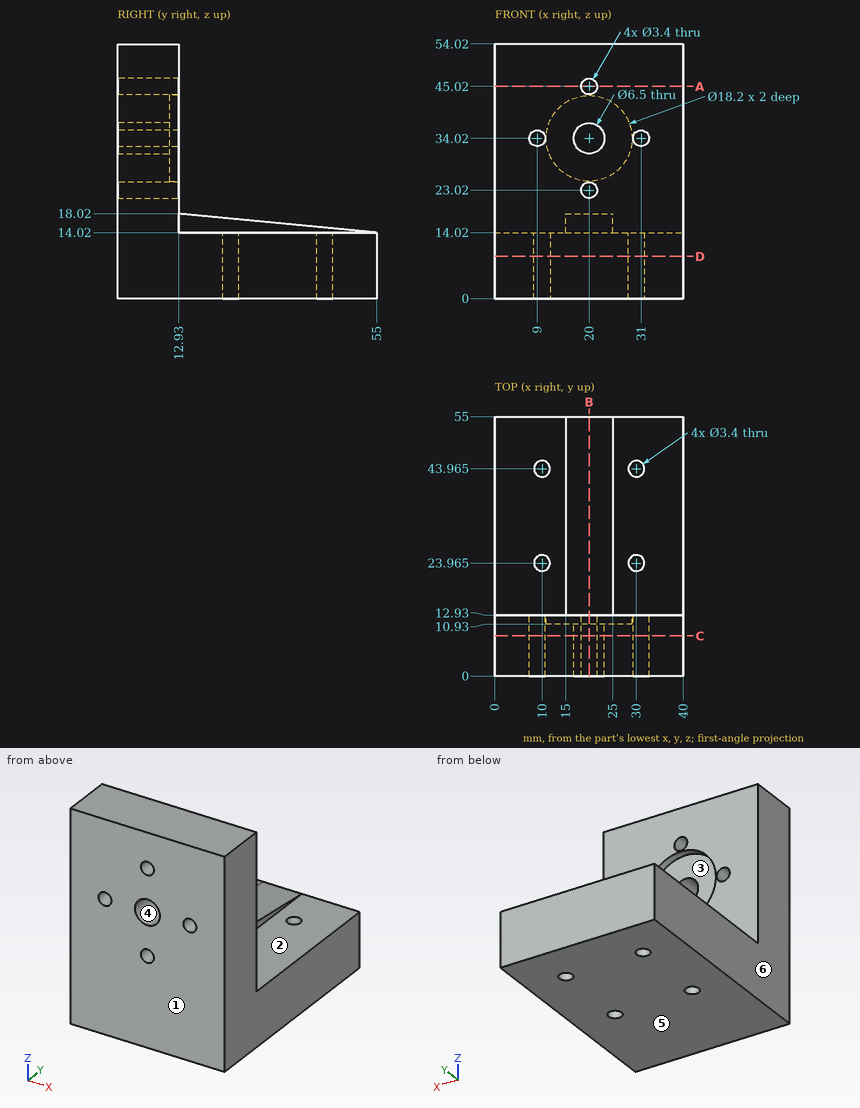
Design review of the part shown in the three views and the two pictorial views. Dimensions are in mm from the part's minimum x, y and z. A direction names the side the tool comes from. Round coordinates to 2 decimals unless told otherwise and drop trailing zeros. Write each loop counter-clockwise with the first axis right and the second up, starting at its lowest first coordinate (ties: lowest second). Pieces come first, ordered by that corner, then holes. Notation, with made-up numbers: M 70.25,16.25 L 75.25,16.25 A26 ccw 75.25,35.25 Z; hole C 16,-12 d3. An arc over 180 degrees is marked long. One line per item, written item: value. Start each with the question number.
1. For the marked faces 1, 2 and 3, list the 3-axis set-ups (+Z, -Z, +X, -X, +Y, -Y) from which the entire face can be reached by the end or side of a thin tool; tool diameter is ignored.
2. To check wall thickness, follow probe 1 along Y at (x, z) = (30, 8) (3 decimals); probe 2 along X at (y, z) = (5.25, 45.02); probe 3 along Y at (x, z) = (29.5, 36.5). State the ranges of each line that lie inside material, in increasing order. Write a range as from..to.
3. Clearance check with flat-ended pins moving along their axes: P1, Ø4, axis at x = 19.5, y = 23.5, coming from the +Z side; P2, Ø4, axis at x = 20, z = 23.02, coming from the +Y side; P3, Ø1, axis at x = 21.5, z = 30, coming from the +Y side. State where each tip first meets the part, or that it passes through.
4. Take a section at B-B on x = 20. State the section outline as (y, z) points, then the cut area to 3 significant figures.
5. Take a section at D-D on z = 9. State the section outline as (x, y) points (3 decimals).
6. Take a section at C-C on y = 8.5. State the section outline as (x, z) points, then the cut area to 3 significant figures.
7. Take a section at A-A on z = 45.02. State the section outline as (x, y) points, then the cut area to 3 significant figures.
8. Draft analysis for pull direction X (two halves, no side actions). For the marked faces 4, 5 and 6, state which applies: pulls with the +X half, pulls with the -X half, needs draft (parallel to the pull), parting line crosses it, or undercut.
Computed:
1. face 1: +Z, -Z, +X, -X, -Y
1. face 2: +Z, +X, +Y
1. face 3: +Y
2. probe 1: y = 0..22.265, 25.665..42.265, 45.665..55
2. probe 2: x = 0..18.3, 21.7..40
2. probe 3: y = 0..12.93
3. P1: stops at z = 17.21
3. P2: stops at y = 12.93
3. P3: stops at y = 10.93
4. outline: M 0,0 L 55,0 L 55,14.02 L 12.93,18.02 L 12.93,21.32 L 0,21.32 Z; M 0,24.72 L 12.93,24.72 L 12.93,24.92 L 10.93,24.92 L 10.93,30.77 L 0,30.77 Z; M 0,37.27 L 10.93,37.27 L 10.93,43.12 L 12.93,43.12 L 12.93,43.32 L 0,43.32 Z; M 0,46.72 L 12.93,46.72 L 12.93,54.02 L 0,54.02 Z
4. area: 1,180 mm²
5. outline: M 0,0 L 40,0 L 40,55 L 0,55 Z; hole C 10,23.965 d3.4; hole C 10,43.965 d3.4; hole C 30,23.965 d3.4; hole C 30,43.965 d3.4
6. outline: M 0,0 L 40,0 L 40,54.02 L 0,54.02 Z; hole C 9,34.02 d3.4; hole C 20,34.02 d6.5; hole C 20,23.02 d3.4; hole C 20,45.02 d3.4; hole C 31,34.02 d3.4
6. area: 2,090 mm²
7. outline: M 0,0 L 18.3,0 L 18.3,12.93 L 0,12.93 Z; M 21.7,0 L 40,0 L 40,12.93 L 21.7,12.93 Z
7. area: 473 mm²
8. face 4: undercut
8. face 5: needs draft
8. face 6: pulls with the -X half
